Design review of the part built by this model. Coordinates are the model's own, in mm. Face numbers are marked on the shaded views. Coordinates: 2 decimals unless noted, no trailing zeros. Write each loop counter-clockwise with the first axis right and the second up, starting at its lowest first coordinate (ties: lowest second). Pieces come first, ordered by that corner, then holes.
Q1. Add section A-A, the plane y = 0. Give the boundary of the cut face in (x, z), plus the area to 3 significant figures.
Q2. Add section B-B, the plane x = -65.5. Give the boundary of the cut face in (y, z).
Q3. Add section D-D, the plane x = -16. Give the boundary of the cut face in (y, z), plus the area to 3 significant figures.
Q4. Add section C-C, the plane z = 121. Give the boundary of the cut face in (x, y), plus the area to 3 significant figures.
Q5. Clearance check with flat-ended pins moving along their axes: pin 1 Ø10 at (x, y) = (-68, -14.5) entering from +Z; pin 2 Ø20.5 at (x, z) = (-39, 50) entering from -Y; pin 3 Ø12.5 at (x, z) = (-35.5, 53) entering from +Y. State where each tip first meets the part, or that it passes through.
Q6. The part is to be moulded in two halves that separate along Y. For the marked faces 1, 2 and 3, say which applies: +Y half, -Y half, draft (parallel to the pull), parting line (faces both ways), or undercut.
Q7. To check wall thickness, follow probe 1 along Y at (x, z) = (-7.5, 114.3); probe 2 along Z at (x, y) = (-15, 0); probe 3 along Z at (x, y) = (-23.75, 0). State the ranges of each line that lie inside material, in increasing order.
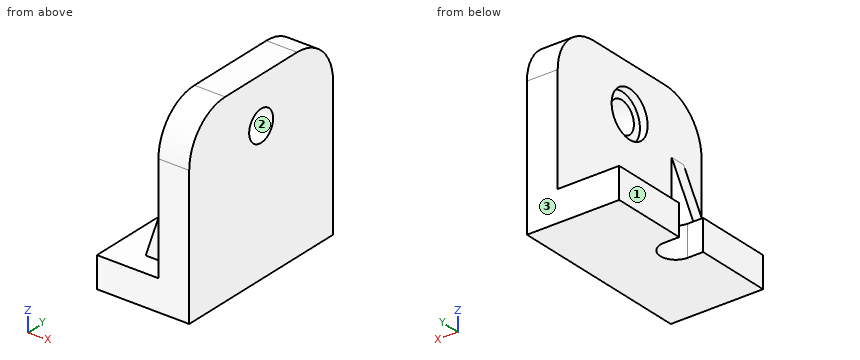
from build123d import *

# Parameters (mm, degrees)
F1_DEPTH  = 76.2
F2_R      = 12.7
F3_DEPTH  = 76.201
F5_DEPTH  = 25.401
F7_DEPTH  = 25.401
F8_R      = 19.05
F8_R_2    = 12.7
F9_DEPTH  = 6.35
F12_DEPTH = 12.7


with BuildPart() as f1:
    # F0 (on Front) → F1 (new body, symmetric)
    with BuildSketch(Plane.XZ):
        Polygon((0, 0), (0, 152.4), (-25.4, 152.4), (-25.4, 25.4), (-76.2, 25.4), (-76.2, 0), align=None)
    extrude(amount=F1_DEPTH, both=True)

    # F2 (on face) → F3 (cut, through all)
    with BuildSketch(Plane.YZ):
        with Locations((0, 114.3)):
            Circle(F2_R)
    extrude(amount=-F3_DEPTH, mode=Mode.SUBTRACT)

    # F4 (on face) → F5 (cut, through all)
    with BuildSketch(Plane.XY.offset(25.4)):
        with BuildLine():
            Line((-76.2, 12.7), (-76.2, -12.7))
            Line((-76.2, -12.7), (-63.5, -12.7))
            ThreePointArc((-63.5, -12.7), (-50.8, 0), (-63.5, 12.7))
            Line((-63.5, 12.7), (-76.2, 12.7))
        make_face()
    extrude(amount=-F5_DEPTH, mode=Mode.SUBTRACT)

    # F6 (on face) → F7 (cut, through all)
    with BuildSketch(Plane(origin=(-25.4, 0, 0), x_dir=(0, -1, 0), z_dir=(-1, 0, 0))):
        with BuildLine():
            Line((-76.2, 152.4), (-76.2, 114.3))
            ThreePointArc((-76.2, 114.3), (-65.0407683632, 141.2407683632), (-38.1, 152.4))
            Line((-38.1, 152.4), (-76.2, 152.4))
        make_face()
        with BuildLine():
            ThreePointArc((38.1, 152.4), (65.0407683632, 141.2407683632), (76.2, 114.3))
            Line((76.2, 114.3), (76.2, 152.4))
            Line((76.2, 152.4), (38.1, 152.4))
        make_face()
    extrude(amount=-F7_DEPTH, mode=Mode.SUBTRACT)

    # F8 (on face) → F9 (cut)
    with BuildSketch(Plane(origin=(-25.4, 0, 0), x_dir=(0, -1, 0), z_dir=(-1, 0, 0))):
        with Locations((0, 114.3)):
            Circle(F8_R)
        with Locations((0, 114.3)):
            Circle(F8_R_2, mode=Mode.SUBTRACT)
    extrude(amount=-F9_DEPTH, mode=Mode.SUBTRACT)

    # F11 (on offset) → F12 (join)
    with BuildSketch(Plane.XZ.offset(44.45)):
        Polygon((-25.4, 101.6), (-50.8, 25.4), (-25.4, 25.4), align=None)
    extrude(amount=F12_DEPTH)


solid = f1.part
Here are the results:
1. outline: (-50.8, 0) - (0, 0) - (0, 101.6) - (-19.05, 101.6) - (-19.05, 95.25) - (-25.4, 95.25) - (-25.4, 25.4) - (-50.8, 25.4) - close; (-25.4, 133.35) - (-19.05, 133.35) - (-19.05, 127) - (0, 127) - (0, 152.4) - (-25.4, 152.4) - close
1. area: 3,790 mm2
2. outline: (-76.2, 0) - (-12.7, 0) - (-12.7, 25.4) - (-76.2, 25.4) - close; (12.7, 0) - (76.2, 0) - (76.2, 25.4) - (12.7, 25.4) - close
3. outline: (-76.2, 0) - (76.2, 0) - (76.2, 114.3) arc R38.1 ccw to (38.1, 152.4) - (-38.1, 152.4) arc R38.1 ccw to (-76.2, 114.3) - close; hole circle Ø25.4 at (0, 114.3)
3. area: 22,100 mm2
4. outline: (-25.4, -75.61) - (0, -75.61) - (0, -10.79) - (-19.05, -10.79) - (-19.05, -17.83) - (-25.4, -17.83) - close; (-25.4, 17.83) - (-19.05, 17.83) - (-19.05, 10.79) - (0, 10.79) - (0, 75.61) - (-25.4, 75.61) - close
4. area: 3,200 mm2
5. pin 1: stops at z = 25.4
5. pin 2: stops at y = -57.15
5. pin 3: stops at y = -44.45
6. face 1: draft
6. face 2: undercut
6. face 3: +Y half
7. probe 1: y = -76.2 to -12.7, 12.7 to 76.2
7. probe 2: z = 0 to 101.6, 127 to 152.4
7. probe 3: z = 0 to 95.25, 133.35 to 152.4
